```python
from build123d import *
from build123d.topology import SkipClean

# Parameters (mm, degrees)
SKETCH1_R          = 2.778125
SKETCH1_R_2        = 8.382
EXTRUDE1_DEPTH     = 1.5875
CUT_EXTRUDE2_DEPTH = 33.32239767
SKETCH4_R          = 3.4925
CUT_EXTRUDE3_DEPTH = 0.508
CUT_EXTRUDE4_START = -0.508
SKETCH5_R          = 3.4925
CUT_EXTRUDE4_DEPTH = 0.508


with BuildPart() as part:
    # Sketch1 → Extrude1 (new body)
    with BuildSketch(Plane.XY):
        with BuildLine():
            Line((-22.362691327, 6.521593303), (-6.155612245, 13.767808085))
            ThreePointArc((-6.155612245, 13.767808085), (0, 15.08125), (6.155612245, 13.767808085))
            Line((6.155612245, 13.767808085), (22.362691327, 6.521593303))
            ThreePointArc((22.362691327, 6.521593303), (26.590625, 0), (22.362691327, -6.521593303))
            Line((22.362691327, -6.521593303), (6.155612245, -13.767808085))
            ThreePointArc((6.155612245, -13.767808085), (0, -15.08125), (-6.155612245, -13.767808085))
            Line((-6.155612245, -13.767808085), (-22.362691327, -6.521593303))
            ThreePointArc((-22.362691327, -6.521593303), (-26.590625, 0), (-22.362691327, 6.521593303))
        make_face()
        with Locations((-19.446875, 0)):
            Circle(SKETCH1_R, mode=Mode.SUBTRACT)
        with Locations((19.446875, 0)):
            Circle(SKETCH1_R, mode=Mode.SUBTRACT)
        Circle(SKETCH1_R_2, mode=Mode.SUBTRACT)
    extrude(amount=EXTRUDE1_DEPTH)

    # Sketch2 → Revolve1 (revolve)
    with BuildSketch(Plane(origin=(0, 0, 0), x_dir=(0, 0, -1), z_dir=(1, 0, 0))):
        with BuildLine():
            Line((0, 8.382), (-1.5875, 8.382))
            Line((-1.5875, 8.382), (-11.53560961, 7.860641667))
            ThreePointArc((-11.53560961, 7.860641667), (-11.798841313, 7.73929019), (-11.90625, 7.47006819))
            ThreePointArc((-11.90625, 7.47006819), (-11.791696686, 7.193512026), (-11.515140521, 7.078958711))
            Line((-11.515140521, 7.078958711), (-10.499140521, 7.078958711))
            Line((-10.499140521, 7.078958711), (-10.499140521, 6.102969034))
            Line((-10.499140521, 6.102969034), (-11.39825, 6.102969034))
            Line((-11.39825, 6.102969034), (-11.39825, 5.126979356))
            Line((-11.39825, 5.126979356), (-10.499140521, 5.126979356))
            Line((-10.499140521, 5.126979356), (-10.499140521, 4.150989678))
            Line((-10.499140521, 4.150989678), (-10.499140521, 3.175))
            Line((-10.499140521, 3.175), (0, 3.175))
            Line((0, 3.175), (0, 8.382))
        make_face()
    revolve(axis=Axis((0, 0, 0), (0, 0, 1)))

    # Sketch3 → Cut-Extrude2 (cut, through all)
    with BuildSketch(Plane.XY.offset(10.499140521)):
        with BuildLine():
            ThreePointArc((-1.624027636, 3.0919396), (-1.940329039, 2.903907621), (-2.235091242, 2.683639952))
            ThreePointArc((-2.235091242, 2.683639952), (-2.24506403, 2.24506403), (-2.683639952, 2.235091242))
            ThreePointArc((-2.683639952, 2.235091242), (-2.903907621, 1.940329039), (-3.0919396, 1.624027636))
            ThreePointArc((-3.0919396, 1.624027636), (-2.933317516, 1.215019898), (-3.334692412, 1.037970504))
            ThreePointArc((-3.334692412, 1.037970504), (-3.425392592, 0.68135295), (-3.478068182, 0.317171835))
            ThreePointArc((-3.478068182, 0.317171835), (-3.175, 0), (-3.478068182, -0.317171835))
            ThreePointArc((-3.478068182, -0.317171835), (-3.425392592, -0.68135295), (-3.334692412, -1.037970504))
            ThreePointArc((-3.334692412, -1.037970504), (-2.933317516, -1.215019898), (-3.0919396, -1.624027636))
            ThreePointArc((-3.0919396, -1.624027636), (-2.903907621, -1.940329039), (-2.683639952, -2.235091242))
            ThreePointArc((-2.683639952, -2.235091242), (-2.24506403, -2.24506403), (-2.235091242, -2.683639952))
            ThreePointArc((-2.235091242, -2.683639952), (-1.940329039, -2.903907621), (-1.624027636, -3.0919396))
            ThreePointArc((-1.624027636, -3.0919396), (-1.215019898, -2.933317516), (-1.037970504, -3.334692412))
            ThreePointArc((-1.037970504, -3.334692412), (-0.68135295, -3.425392592), (-0.317171835, -3.478068182))
            ThreePointArc((-0.317171835, -3.478068182), (0, -3.175), (0.317171835, -3.478068182))
            ThreePointArc((0.317171835, -3.478068182), (0.68135295, -3.425392592), (1.037970504, -3.334692412))
            ThreePointArc((1.037970504, -3.334692412), (1.215019898, -2.933317516), (1.624027636, -3.0919396))
            ThreePointArc((1.624027636, -3.0919396), (1.940329039, -2.903907621), (2.235091242, -2.683639952))
            ThreePointArc((2.235091242, -2.683639952), (2.24506403, -2.24506403), (2.683639952, -2.235091242))
            ThreePointArc((2.683639952, -2.235091242), (2.903907621, -1.940329039), (3.0919396, -1.624027636))
            ThreePointArc((3.0919396, -1.624027636), (2.933317516, -1.215019898), (3.334692412, -1.037970504))
            ThreePointArc((3.334692412, -1.037970504), (3.425392592, -0.68135295), (3.478068182, -0.317171835))
            ThreePointArc((3.478068182, -0.317171835), (3.175, 0), (3.478068182, 0.317171835))
            ThreePointArc((3.478068182, 0.317171835), (3.425392592, 0.68135295), (3.334692412, 1.037970504))
            ThreePointArc((3.334692412, 1.037970504), (2.933317516, 1.215019898), (3.0919396, 1.624027636))
            ThreePointArc((3.0919396, 1.624027636), (2.903907621, 1.940329039), (2.683639952, 2.235091242))
            ThreePointArc((2.683639952, 2.235091242), (2.24506403, 2.24506403), (2.235091242, 2.683639952))
            ThreePointArc((2.235091242, 2.683639952), (1.940329039, 2.903907621), (1.624027636, 3.0919396))
            ThreePointArc((1.624027636, 3.0919396), (1.215019898, 2.933317516), (1.037970504, 3.334692412))
            ThreePointArc((1.037970504, 3.334692412), (0.68135295, 3.425392592), (0.317171835, 3.478068182))
            ThreePointArc((0.317171835, 3.478068182), (0, 3.175), (-0.317171835, 3.478068182))
            ThreePointArc((-0.317171835, 3.478068182), (-0.68135295, 3.425392592), (-1.037970504, 3.334692412))
            ThreePointArc((-1.037970504, 3.334692412), (-1.215019898, 2.933317516), (-1.624027636, 3.0919396))
        make_face()
    extrude(amount=-CUT_EXTRUDE2_DEPTH, mode=Mode.SUBTRACT)

    # Sketch4 → Cut-Extrude3 (cut)
    with BuildSketch(Plane.XY.offset(10.499140521)):
        Circle(SKETCH4_R)
    extrude(amount=-CUT_EXTRUDE3_DEPTH, mode=Mode.SUBTRACT)

    # Sketch5 → Cut-Extrude4 (cut)
    with SkipClean():  # the faces are left unmerged after this step: merging them gives an invalid solid
        with BuildSketch(Plane(origin=(0, 0, 0), x_dir=(-1, 0, 0), z_dir=(0, 0, -1)).offset(CUT_EXTRUDE4_START)):
            with Locations(Location((0, 0, 0), (0, 0, 180))):
                Circle(SKETCH5_R)
        extrude(amount=CUT_EXTRUDE4_DEPTH, mode=Mode.SUBTRACT)


solid = part.part
```
Geometry check sheet. Reference: the model listing, model coordinates, mm. A direction names the side the tool comes from. Give positions to 0.01 mm unless a question says otherwise; leave off trailing zeros. Loops run counter-clockwise (first coordinate to the right, second up) from the corner with the lowest first, then second, coordinate; pieces in that order, holes last. Notation, with made-up numbers: (40, 58) - (91, 58) arc R20 cw to (91, 95) - close; hole circle Ø8 at (7.25, -8.5). An arc over 180 degrees is marked (long way). Use CSV: the item, a comma, the result in double quotes. Start each with the question number.
Q1. Go/stop test with flat-tipped pins: pin 1 Ø2 at (y, z) = (8, 7) entering from +X; pin 2 Ø0.5 at (x, y) = (1.5, 3) entering from +Z; pin 3 Ø1.5 at (y, z) = (8, 9) entering from -X; pin 4 Ø2 at (x, y) = (-0.5, 0.5) entering from +Z. Record where each tip stops, or that it passes through.
Q2. Scan lines: probe 1 along Y at (x, z) = (0, 11); probe 2 along Z at (x, y) = (6.5, -11.5); probe 3 along X at (y, z) = (0, 11.2). Record each from-to range of solid material in increasing order. Write a range as from..to.
Q3. Release check for a two-part mould opening along X. For faces 3 (the face through (3.3, 2.2, 10.499)), 4 (the face through (-14.146, -10.195, 0.783)), 5 (the face through (-0.09, 15.08, 0.78)), 6 (the face through (-6, 2, 10.499)) record: +X half, -X half, draft (parallel to the pull), parting line (faces both ways), or undercut.
Q4. Section check C-C, the plane y = -11. Record the cut outline in (x, z).
Q5. Section check B-B, the plane x = -15. Record the cut outline in (y, z), and give its area (3 significant figures).
Q6. Access from +Z, -Z, +X, -X, +Y, -Y to the whole of each face (thin tool, end or side, straight path). Record for faces 1 (the face through (5.96, -1.32, 10.95)), 2 (the face through (0, 4, 0)).
Findings below:
1,pin 1,"stops at x = 4.08"
1,pin 2,"stops at z = 10.5"
1,pin 3,"stops at x = -3.37"
1,pin 4,"passes through"
2,probe 1,"y = -7.89..-7.08, -6.1..-5.13, 5.13..6.1, 7.08..7.89"
2,probe 2,"z = 0..1.59"
2,probe 3,"x = -7.88..-7.08, -6.1..-5.13, 5.13..6.1, 7.08..7.88"
3,face 3,"undercut"
3,face 4,"-X half"
3,face 5,"parting line"
3,face 6,"undercut"
4,outline,"(-12.35, 0) - (12.35, 0) - (12.35, 1.59) - (-12.35, 1.59) - close"
5,outline,"(-9.81, 0) - (9.81, 0) - (9.81, 1.59) - (-9.81, 1.59) - close"
5,area,"31.2 mm^2"
6,face 1,"+Z"
6,face 2,"-Z, +X, -X, +Y, -Y"
